Design review of the part shown in the three views and the two pictorial views. Dimensions are in mm from the part's minimum x, y and z. Coordinates: 2 decimals unless noted, no trailing zeros. Order: outer loops, then holes, each group sorted by start corner. A loop starts at its lowest first (then second) coordinate and runs counter-clockwise, first axis right, second up. Notation, with made-up numbers: (-32, 32) - (6, 32) arc R22 ccw to (6, 65) - close; hole circle Ø7 at (49.25, 24.25). An arc over 180 degrees is marked (long way). One line per item, written item: value. Start each with the question number.
(1) Consider section A-A on z = 7.5. Write out the cut boundary in (x, y), then the cut area to 3 significant figures.
(2) Consider section B-B on x = 67.7. Write out the cut boundary in (y, z).
(3) To check wall thickness, follow line 1 along Z through (x, y) = (60.6, 0.8); line 2 along Z through (x, y) = (73, 2.1); line 3 along X through (y, z) = (3.3, 54.5). State the ranges of each line that lie inside material, in increasing order.
(4) Clearance check with flat-ended pins moving along their axes: pin 1 (1.2 mm diameter, centred on x = 53, y = 4, fed in from -Z); pin 2 (1.2 mm diameter, centred on y = 4.5, z = 52.5, fed in from +X); pin 3 (12 mm diameter, centred on x = 24, z = 15.5, fed in from +Y). State where each tip first meets the part, or that it passes through.
(5) Consider section C-C on y = 3.4. Write out the cut boundary in (x, z).
(6) Mouldability with a two-part tool opening along Z and no side actions: class the marked faces 1 and 2 as released by +Z, released by -Z, zero draft, split by the parting line, or undercut.
(7) Consider section D-D on z = 47.4. Write out the cut boundary in (x, y), then the cut area to 3 significant figures.
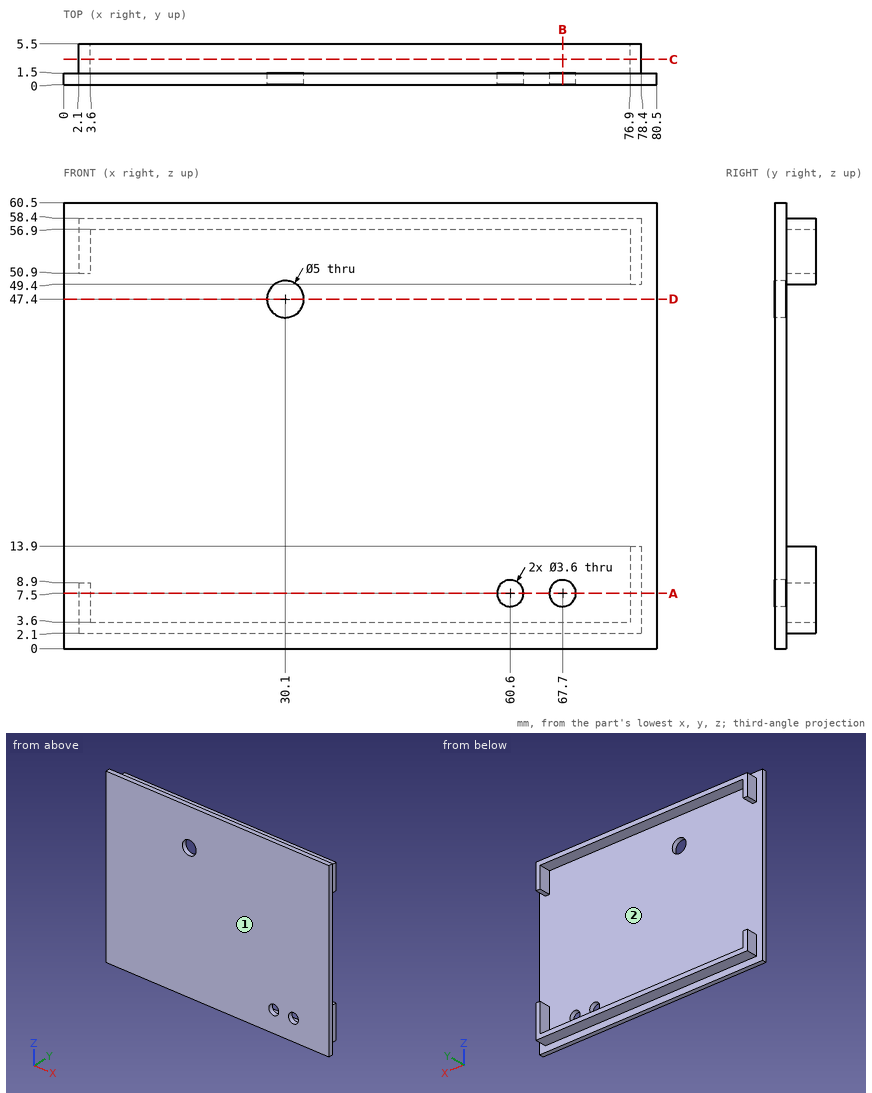
Geometry check:
1. outline: (0, 0) - (58.8, 0) - (58.8, 1.5) - (3.6, 1.5) - (3.6, 5.5) - (2.1, 5.5) - (2.1, 1.5) - (0, 1.5) - close; (62.4, 0) - (65.9, 0) - (65.9, 1.5) - (62.4, 1.5) - close; (69.5, 0) - (80.5, 0) - (80.5, 1.5) - (78.4, 1.5) - (78.4, 5.5) - (76.9, 5.5) - (76.9, 1.5) - (69.5, 1.5) - close
1. area: 122 mm^2
2. outline: (0, 0) - (1.5, 0) - (1.5, 2.1) - (5.5, 2.1) - (5.5, 3.6) - (1.5, 3.6) - (1.5, 5.7) - (0, 5.7) - close; (0, 9.3) - (1.5, 9.3) - (1.5, 56.9) - (5.5, 56.9) - (5.5, 58.4) - (1.5, 58.4) - (1.5, 60.5) - (0, 60.5) - close
3. line 1: z = 0 to 5.7, 9.3 to 60.5
3. line 2: z = 2.1 to 3.6, 56.9 to 58.4
3. line 3: x = 2.1 to 3.6, 76.9 to 78.4
4. pin 1: stops at z = 2.1
4. pin 2: stops at x = 78.4
4. pin 3: stops at y = 1.5
5. outline: (2.1, 2.1) - (78.4, 2.1) - (78.4, 13.9) - (76.9, 13.9) - (76.9, 3.6) - (3.6, 3.6) - (3.6, 8.9) - (2.1, 8.9) - close; (2.1, 50.9) - (3.6, 50.9) - (3.6, 56.9) - (76.9, 56.9) - (76.9, 49.4) - (78.4, 49.4) - (78.4, 58.4) - (2.1, 58.4) - close
6. face 1: zero draft
6. face 2: undercut
7. outline: (0, 0) - (27.6, 0) - (27.6, 1.5) - (0, 1.5) - close; (32.6, 0) - (80.5, 0) - (80.5, 1.5) - (32.6, 1.5) - close
7. area: 113 mm^2
